Autodesk Inventor part; units mm, degrees
ref_plane "YZ Plane" through (0, 0, 0) normal (1, 0, 0) x (0, 1, 0)
ref_plane "XZ Plane" through (0, 0, 0) normal (0, 1, 0) x (-1, 0, 0)
ref_plane "XY Plane" through (0, 0, 0) normal (0, 0, 1) x (1, 0, 0)
sketch "Sketch1" plane through (0, 0, 0) normal (0, 1, 0) x (-1, 0, 0)
  circle A0 centre (0, 0) radius 15
  dimension "d0" = 30
extrude "Extrusion1" add sketch "Sketch1" along normal blind 3
sketch "Sketch2" plane through (0, 3, 0) normal (0, 1, 0) x (1, 0, 0)
  circle A0 centre (0, 0) radius 12 construction
  point P0 (0, 12)
  point P1 (-10.3923, -6)
  point P2 (10.3923, -6)
  dimension "d3" = 24
  dimension "d4" = 120
hole "Hole1" at (0, 3, -12) at (-10.3923, 3, 6) at (10.3923, 3, 6) direction (0, -1, 0) diameter 3.2 end through all
sketch "Sketch4" plane through (0, 3, 0) normal (0, 1, 0) x (1, 0, 0)
  circle A0 centre (0, -12) radius 3.5
  circle A1 centre (0, 0) radius 15
  arc A2 (-3.5, -14.586) -> (3.5, -14.586) centre (0, 0) ccw
  line L0 (3.5, -12) -> (3.5, -14.586)
  line L1 (-3.5, -12) -> (-3.5, -14.586)
  dimension "d12" = 7
  dimension "d13" = 12
extrude "Extrusion2" cut sketch "Sketch4" against normal through all contours A0 A1 | L0 A1 A0 | A0 A1 L1 picked at (0.1406, -12.8318)
pattern_circular "Circular Pattern1" count 3 over 360 about axis through (0, 0, 0) along (0, 1, 0) of "Extrusion2"
sketch "Sketch6" plane through (0, 3, 0) normal (0, 1, 0) x (1, 0, 0)
  circle A0 centre (0, 0) radius 3
  dimension "d24" = 6
extrude "Extrusion4" add sketch "Sketch6" along normal blind 12
sketch "Sketch7" plane through (0, 0, 0) normal (0, -1, 0) x (1, 0, 0)
  line L0 (-1.5, 0) -> (63.9289, 0) construction
  line L1 (0, -1.5) -> (62.4289, -1.5)
  line L2 (62.4289, 1.5) -> (0, 1.5)
  arc A0 (0, 1.5) -> (0, -1.5) centre (0, 0) ccw
  arc A1 (62.4289, -1.5) -> (62.4289, 1.5) centre (62.4289, 0) ccw
  point P0 (31.2144, 0)
  dimension "d27" = 3
extrude "Extrusion5" [suppressed]
sketch "Sketch8" plane through (0, 15, 0) normal (0, 1, 0) x (1, 0, 0)
  point P0 (0, 0)
  point P1 (0, 0)
hole "Hole2" at (0, 15, 0) direction (0, -1, 0) diameter 3.242 end through all
sketch "Sketch9" plane through (0, 0, 0) normal (0, -1, 0) x (1, 0, 0)
  arc A0 (12.1423, -2.9689) -> (8.6423, -9.0311) centre (10.3923, -6) ccw
  line L0 (0, 0) -> (10.3923, -6) construction
  line L1 (0, 0) -> (9.8835, -17.1187) construction
  line L2 (0, 0) -> (17.8778, 0) construction
  line L3 (19.4334, 1) -> (1.2758, 1)
  circle A1 centre (0, 0) radius 1.621
  line L4 (-0.2281, -1.6049) -> (7.499, -14.9886)
  arc A2 (-10.8818, -10.3241) -> (10.8818, -10.3241) centre (0, 0) ccw
  arc A3 (14.3818, -4.2619) -> (3.5, 14.586) centre (0, 0) ccw
  arc A4 (6.6173, -13.4615) -> (14.9666, 1) centre (0, 0) ccw
  point P0 (10.8818, -10.3241)
  point P1 (14.3818, -4.2619)
  dimension "d37" = 30
  dimension "d38" = 30
  dimension "d39" = 1
  dimension "d40" = 1
extrude "Extrusion6" cut sketch "Sketch9" against normal blind 10 contours A3 A4 A2 L4 A1 L3
fillet "Fillet1" radius 1 6 edges at (14.9666, 1.5, 1) (6.6173, 1.5, -13.4615) (-3.5, 1.5, 14.586) (3.5, 1.5, 14.586) (-14.3818, 1.5, -4.2619) (-10.8818, 1.5, -10.3241)
equation "\"d38\" = d37"
equation "\"d40\" = d39"
properties part number "FrameSupport-Flange-Slit" material "Copper"
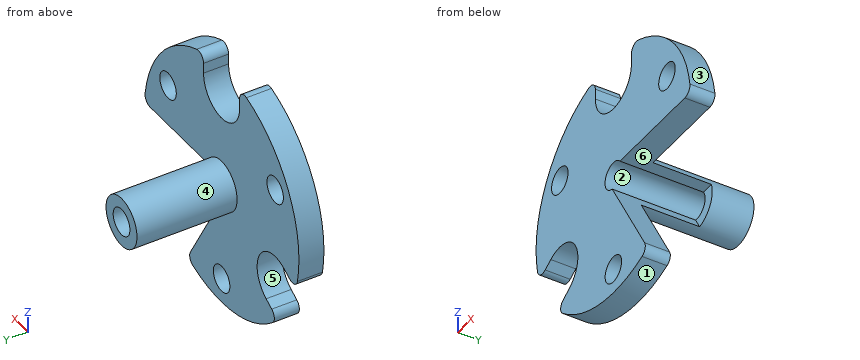
Work out the finished part from the listing and answer in its coordinate system (mm). Face numbers are marked on the shaded views. A direction names the side the tool comes from. Coordinates: 2 decimals unless noted, no trailing zeros. Loops run counter-clockwise (first coordinate to the right, second up) from the corner with the lowest first, then second, coordinate; pieces in that order, holes last. Notation, with made-up numbers: (15.25, 88.5) -> (34.25, 88.5) arc R25 cw to (34.25, 108.5) -> close; hole circle Ø6 at (-17.5, 62). An arc over 180 degrees is marked (long way). Answer as CSV lines item,"result".
Q1. The part is cut by section B-B on x = 9.25. Write down the section's boundary in (y, z), and give its area (3 significant figures).
Findings:
outline,"(0, 1) -> (3, 1) -> (3, 4.88) -> (0, 4.88) -> close; (0, 7.12) -> (3, 7.12) -> (3, 11.81) -> (0, 11.81) -> close"
area,"25.7 mm²"
Q2. The part is cut by section C-C on z = 5.5. Write down the section's boundary in (x, y), and give its area (3 significant figures).
Findings:
outline,"(-13.96, 0) -> (-11.91, 0) -> (-11.91, 3) -> (-13.96, 3) -> close; (-8.87, 0) -> (8.87, 0) -> (8.87, 3) -> (-8.87, 3) -> close; (11.91, 0) -> (13.96, 0) -> (13.96, 3) -> (11.91, 3) -> close"
area,"65.5 mm²"
Q3. The part is cut by section D-D on y = 14.25. Write down the section's boundary in (x, z).
Findings:
outline,"circle Ø6 at (0, 0); hole circle Ø3.24 at (0, 0)"
Q4. A tool of negligible diameter and unlimited length cuts with its end or side. For the marked faces 5 and 6, from which of +Z, -Z, +X, -X, +Y, -Y can it reach the whole face along a straight path? Write none if from no direction.
Findings:
face 5,"+Y, -Y"
face 6,"+X, -Y"
Q5. For a pull along Z with two mould halves and no side action, classify the marked faces 1, 2, 3 and 4 as +Z half, -Z half, draft (parallel to the pull), parting line (faces both ways), or undercut.
Findings:
face 1,"-Z half"
face 2,"undercut"
face 3,"+Z half"
face 4,"parting line"
Q6. Each of these flat-tipped pins is pushed along its axis until it touches: pin 1 (1 mm diameter, centred on y = 1.5, z = 13, fed in from +X); pin 2 (1.4 mm diameter, centred on y = 1, z = 13, fed in from -X); pin 3 (3.5 mm diameter, centred on x = 0, z = -12, fed in from +Y). Where does it stop, or does it pass through?
Findings:
pin 1,"stops at x = 8.29"
pin 2,"stops at x = -8.59"
pin 3,"stops at y = 3"
Q7. The part is cut by section A-A on z = 0. Write down the section's boundary in (x, y), and give its area (3 significant figures).
Findings:
outline,"(-15, 0) -> (-1.62, 0) -> (-1.62, 15) -> (-3, 15) -> (-3, 3) -> (-15, 3) -> close; (1.62, 10) -> (3, 10) -> (3, 15) -> (1.62, 15) -> close"
area,"63.6 mm²"
Q8. Find the intervals of material crossed by probe 1 along Z at (x, y) = (0, 1.4); probe 2 along Y at (x, z) = (9, 8.75); probe 3 along X at (y, z) = (2.1, 6), in increasing order.
Findings:
probe 1,"z = -15 to -13.6, -10.4 to -2, 1.62 to 8.5"
probe 2,"y = 0 to 3"
probe 3,"x = -13.75 to -11.99, -8.79 to 8.79, 11.99 to 13.75"
